Check sheet for the modelled part. Datum: model origin and axes. Units: mm. Face numbers are marked on the shaded views. A direction names the side the tool comes from. Give positions to 0.01 mm unless a question says otherwise; leave off trailing zeros. Loops run counter-clockwise (first coordinate to the right, second up) from the corner with the lowest first, then second, coordinate; pieces in that order, holes last. Notation, with made-up numbers: (5.5, 6.25) -> (23.5, 6.25) arc R25 ccw to (23.5, 26.25) -> close; hole circle Ø11 at (74, 80.5). An arc over 180 degrees is marked (long way). Write each question's results on one line, items separated by ' | '. Start each with the question number.
Item 1: Cross-section at B-B on x = -28. Enter the section's corners in (y, z) (3 decimals), then the cut area to 3 significant figures.
Item 2: Scan lines: line 1 along Z through (x, y) = (-28, 3.2); line 2 along X through (y, z) = (10, 2.5); line 3 along X through (y, z) = (5.5, 1.5). Record each from-to range of solid material in increasing order.
Item 3: Cross-section at C-C on z = 6. Enter the section's corners in (x, y) (3 decimals), then the cut area to 3 significant figures.
Item 4: Access from +Z, -Z, +X, -X, +Y, -Y to the whole of each face (thin tool, end or side, straight path). Record for the marked faces 1, 2 and 3.
Item 5: Cross-section at A-A on z = 0. Enter the section's corners in (x, y).
Item 6: Cross-section at D-D on y = 2.25. Enter the section's corners in (x, z), then the cut area to 3 significant figures.
Item 7: Gauge pin test, flat ends, axial feed: pin 1 Ø11 at (x, z) = (1.5, 2) entering from -Y; pin 2 Ø8 at (x, z) = (28, -10) entering from -Y. Record the tip position at first contact, or that the pin passes through.
Item 8: Mould release check, pull along X, two halves, no side actions. Record for the marked faces 4, 5 and 6: pulls with the +X half, pulls with the -X half, needs draft (parallel to the pull), parting line crosses it, or undercut.
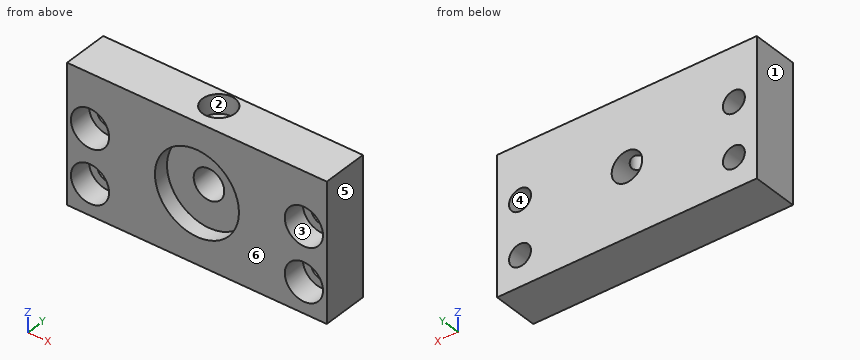
from build123d import *

# Parameters (mm, degrees)
SKETCH1_W           = 68
SKETCH1_H           = 36
BOSS_EXTRUDE1_DEPTH = 12
SKETCH2_R           = 11
CUT_EXTRUDE1_DEPTH  = 4
SKETCH3_R           = 4
CUT_EXTRUDE2_DEPTH  = 9
CUT_EXTRUDE3_REACH  = 38
SKETCH4_R           = 2.375
CUT_EXTRUDE4_REACH  = 14
SKETCH5_R           = 2.875
SKETCH6_R           = 5
CUT_EXTRUDE5_DEPTH  = 6
SKETCH7_R           = 4.25
CUT_EXTRUDE6_DEPTH  = 5


with BuildPart() as part:
    # Sketch1 → Boss-Extrude1 (new body)
    with BuildSketch(Plane(origin=(0, 0, 0), x_dir=(1, 0, 0), z_dir=(0, 1, 0))):
        Rectangle(SKETCH1_W, SKETCH1_H)
    extrude(amount=BOSS_EXTRUDE1_DEPTH)

    # Sketch2 → Cut-Extrude1 (cut)
    with BuildSketch(Plane.XZ):
        Circle(SKETCH2_R)
    extrude(amount=-CUT_EXTRUDE1_DEPTH, mode=Mode.SUBTRACT)

    # Sketch3 → Cut-Extrude2 (cut, through all)
    with BuildSketch(Plane.XZ.offset(-4)):
        Circle(SKETCH3_R)
    extrude(amount=-CUT_EXTRUDE2_DEPTH, mode=Mode.SUBTRACT)

    # Sketch4 → Cut-Extrude3 (cut, up to next)
    with BuildSketch(Plane.XY.offset(18), mode=Mode.PRIVATE) as cut_extrude3_sk1:
        with Locations((0, 7.25)):
            Circle(SKETCH4_R)
    cut_extrude3_tool1 = extrude(cut_extrude3_sk1.sketch, amount=-CUT_EXTRUDE3_REACH, mode=Mode.PRIVATE) & part.part
    add(cut_extrude3_tool1.solids().sort_by_distance((0, 7.25, 18))[0], mode=Mode.SUBTRACT)

    # Sketch5 → Cut-Extrude4 (cut, up to next)
    with BuildSketch(Plane.XZ, mode=Mode.PRIVATE) as cut_extrude4_sk1:
        with Locations((28, 4)):
            Circle(SKETCH5_R)
    cut_extrude4_tool1 = extrude(cut_extrude4_sk1.sketch, amount=-CUT_EXTRUDE4_REACH, mode=Mode.PRIVATE) & part.part
    add(cut_extrude4_tool1.solids().sort_by_distance((28, 0, 4))[0], mode=Mode.SUBTRACT)
    # Sketch5 → Cut-Extrude4 (cut, up to next)
    with BuildSketch(Plane.XZ, mode=Mode.PRIVATE) as cut_extrude4_sk2:
        with Locations((28, -10)):
            Circle(SKETCH5_R)
    cut_extrude4_tool2 = extrude(cut_extrude4_sk2.sketch, amount=-CUT_EXTRUDE4_REACH, mode=Mode.PRIVATE) & part.part
    add(cut_extrude4_tool2.solids().sort_by_distance((28, 0, -10))[0], mode=Mode.SUBTRACT)
    # Sketch5 → Cut-Extrude4 (cut, up to next)
    with BuildSketch(Plane.XZ, mode=Mode.PRIVATE) as cut_extrude4_sk3:
        with Locations((-28, 4)):
            Circle(SKETCH5_R)
    cut_extrude4_tool3 = extrude(cut_extrude4_sk3.sketch, amount=-CUT_EXTRUDE4_REACH, mode=Mode.PRIVATE) & part.part
    add(cut_extrude4_tool3.solids().sort_by_distance((-28, 0, 4))[0], mode=Mode.SUBTRACT)
    # Sketch5 → Cut-Extrude4 (cut, up to next)
    with BuildSketch(Plane.XZ, mode=Mode.PRIVATE) as cut_extrude4_sk4:
        with Locations((-28, -10)):
            Circle(SKETCH5_R)
    cut_extrude4_tool4 = extrude(cut_extrude4_sk4.sketch, amount=-CUT_EXTRUDE4_REACH, mode=Mode.PRIVATE) & part.part
    add(cut_extrude4_tool4.solids().sort_by_distance((-28, 0, -10))[0], mode=Mode.SUBTRACT)

    # Sketch6 → Cut-Extrude5 (cut)
    with BuildSketch(Plane.XZ):
        with Locations((-28, 4)):
            Circle(SKETCH6_R)
        with Locations((28, 4)):
            Circle(SKETCH6_R)
        with Locations((28, -10)):
            Circle(SKETCH6_R)
        with Locations((-28, -10)):
            Circle(SKETCH6_R)
    extrude(amount=-CUT_EXTRUDE5_DEPTH, mode=Mode.SUBTRACT)

    # Sketch7 → Cut-Extrude6 (cut)
    with BuildSketch(Plane.XY.offset(18)):
        with Locations((0, 7.25)):
            Circle(SKETCH7_R)
    extrude(amount=-CUT_EXTRUDE6_DEPTH, mode=Mode.SUBTRACT)


solid = part.part
Answer sheet:
1) outline: (0, -18) -> (12, -18) -> (12, -12.875) -> (6, -12.875) -> (6, -15) -> (0, -15) -> close; (0, -5) -> (6, -5) -> (6, -7.125) -> (12, -7.125) -> (12, 1.125) -> (6, 1.125) -> (6, -1) -> (0, -1) -> close; (0, 9) -> (6, 9) -> (6, 6.875) -> (12, 6.875) -> (12, 18) -> (0, 18) -> close | area: 243 mm²
2) line 1: z = -18 to -15, -5 to -1, 9 to 18 | line 2: x = -34 to -30.45, -25.55 to -3.12, 3.12 to 25.55, 30.45 to 34 | line 3: x = -34 to -32.33, -23.67 to -3.71, 3.71 to 23.67, 32.33 to 34
3) outline: (-34, 0) -> (-32.583, 0) -> (-32.583, 6) -> (-30.065, 6) -> (-30.065, 12) -> (-34, 12) -> close; (-25.935, 6) -> (-23.417, 6) -> (-23.417, 0) -> (-9.22, 0) -> (-9.22, 4) -> (9.22, 4) -> (9.22, 0) -> (23.417, 0) -> (23.417, 6) -> (25.935, 6) -> (25.935, 12) -> (-25.935, 12) -> close; (30.065, 6) -> (32.583, 6) -> (32.583, 0) -> (34, 0) -> (34, 12) -> (30.065, 12) -> close; hole circle Ø4.75 at (0, 7.25) | area: 565 mm²
4) face 1: +Z, -Z, -X, +Y, -Y | face 2: +Z | face 3: -Y
5) outline: (-34, 0) -> (-31, 0) -> (-31, 6) -> (-25, 6) -> (-25, 0) -> (-11, 0) -> (-11, 4) -> (-4, 4) -> (-4, 12) -> (-34, 12) -> close; (4, 4) -> (11, 4) -> (11, 0) -> (25, 0) -> (25, 6) -> (31, 6) -> (31, 0) -> (34, 0) -> (34, 12) -> (4, 12) -> close
6) outline: (-34, -18) -> (34, -18) -> (34, 18) -> (-34, 18) -> close; hole circle Ø10 at (-28, -10); hole circle Ø10 at (-28, 4); hole circle Ø22 at (0, 0); hole circle Ø10 at (28, -10); hole circle Ø10 at (28, 4) | area: 1,750 mm²
7) pin 1: stops at y = 4 | pin 2: stops at y = 6
8) face 4: undercut | face 5: pulls with the +X half | face 6: needs draft
